The figure shows three views and two pictorial views of one solid part (mm, origin at its lowest corner). Answer the questions. A direction names the side the tool comes from. Coordinates: 2 decimals unless noted, no trailing zeros. Write each loop counter-clockwise with the first axis right and the second up, starting at its lowest first coordinate (ties: lowest second). Pieces come first, ordered by that corner, then holes. Notation, with made-up numbers: M 39.25,-8.5 L 76.25,-8.5 A33 cw 76.25,28.5 Z; hole C -27.75,-13 d10. An arc over 180 degrees is marked long. Answer as CSV lines item,"result".
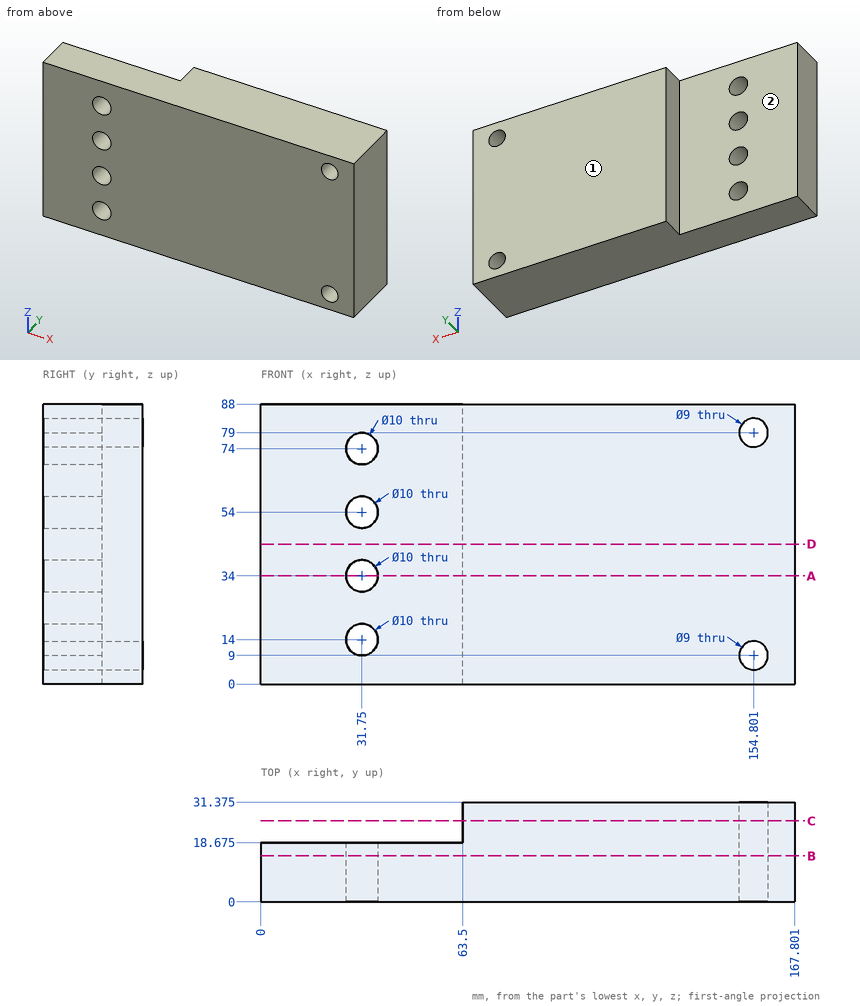
Q1. Find section A-A (z = 34). Give the vertices of the cut face in (x, y) (3 decimals).
Output:
outline,"M 0,0 L 26.75,0 L 26.75,18.675 L 0,18.675 Z; M 36.75,0 L 167.801,0 L 167.801,31.375 L 63.5,31.375 L 63.5,18.675 L 36.75,18.675 Z"
Q2. Straight lines are drawn through the part: line 1 (Z direction, x = 31.75, y = 9.5); line 2 (Z direction, x = 31, y = 6); line 3 (X direction, y = 9, z = 54). For each, find the intervals that lie inside material, in ascending order.
Output:
line 1,"0 to 9, 19 to 29, 39 to 49, 59 to 69, 79 to 88"
line 2,"0 to 9.06, 18.94 to 29.06, 38.94 to 49.06, 58.94 to 69.06, 78.94 to 88"
line 3,"0 to 26.75, 36.75 to 167.8"
Q3. Find section C-C (y = 25.5). Give the vertices of the cut face in (x, z), and give its area (3 significant figures).
Output:
outline,"M 63.5,0 L 167.8,0 L 167.8,88 L 63.5,88 Z; hole C 154.8,9 d9; hole C 154.8,79 d9"
area,"9,050 mm2"
Q4. Flat-ended cylindrical pins translate along their axes: pin 1 Ø10.5 at (x, z) = (154.801, 79) entering from -Y; pin 2 Ø4 at (y, z) = (22.5, 67.5) entering from -X; pin 3 Ø1 at (x, z) = (22.5, 30) entering from +Y (3 decimals). Find the tip coordinate at first contact, or state that the pin passes through.
Output:
pin 1,"y = 0"
pin 2,"x = 63.5"
pin 3,"y = 18.675"
Q5. Find section B-B (y = 14.5). Give the vertices of the cut face in (x, z), and give its area (3 significant figures).
Output:
outline,"M 0,0 L 167.8,0 L 167.8,88 L 0,88 Z; hole C 31.75,14 d10; hole C 31.75,34 d10; hole C 31.75,54 d10; hole C 31.75,74 d10; hole C 154.8,9 d9; hole C 154.8,79 d9"
area,"14,300 mm2"
Q6. Find section D-D (z = 44). Give the vertices of the cut face in (x, y) (3 decimals).
Output:
outline,"M 0,0 L 167.801,0 L 167.801,31.375 L 63.5,31.375 L 63.5,18.675 L 0,18.675 Z"
Q7. For the marked faces 1 and 2, determine the directions among +Z, -Z, +X, -X, +Y, -Y from which every point of the face is accessible in a straight line to the end or side of a thin tool.
Output:
face 1,"+Z, -Z, +X, -X, +Y"
face 2,"+Z, -Z, -X, +Y"
